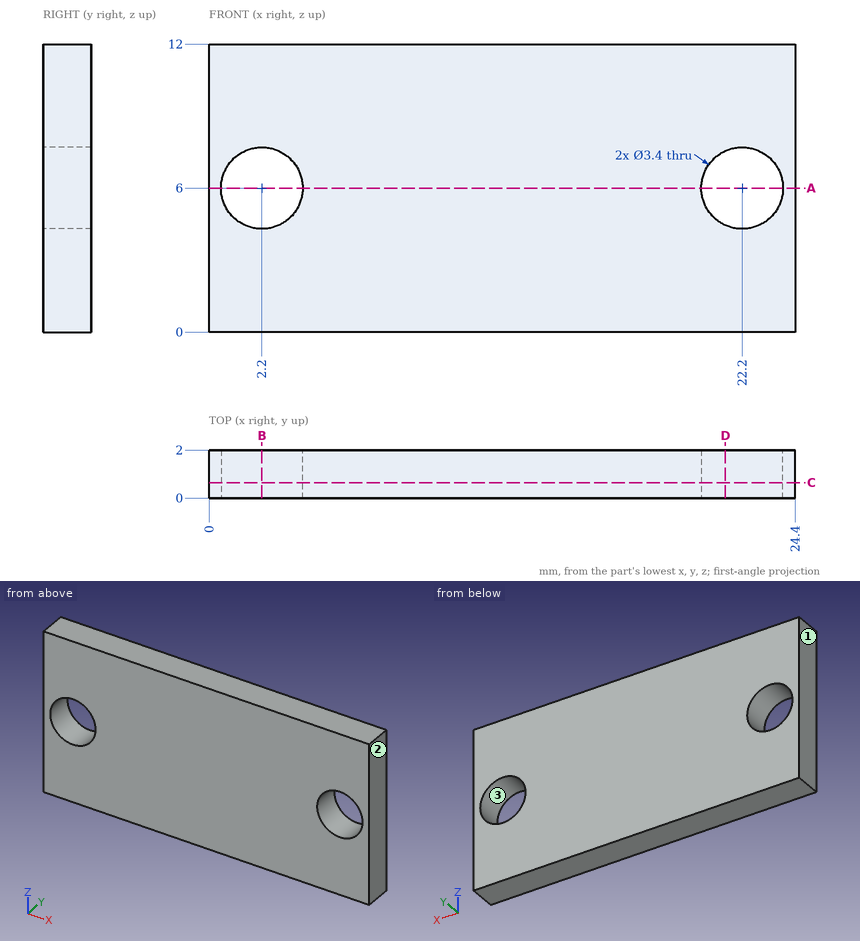
Could you check a few things on this drawing? It's one solid part, dimensions in mm from its lowest x, y, z. Give positions to 0.01 mm unless a question says otherwise; leave off trailing zeros. Write each loop counter-clockwise with the first axis right and the second up, starting at its lowest first coordinate (ties: lowest second). Pieces come first, ordered by that corner, then holes. Notation, with made-up numbers: (81.5, 19) -> (85.5, 19) arc R24 ccw to (85.5, 30) -> close; hole circle Ø1 at (59, 61.5). An arc over 180 degrees is marked (long way). Answer as a JSON object with one key per item and string values.
Q1. We'd pull the mould along X, two halves only. Please class the marked faces 1, 2 and 3: released by +X, released by -X, zero draft, split by the parting line, or undercut.
Taken from the geometry:
{"face 1": "released by -X", "face 2": "released by +X", "face 3": "undercut"}
Q2. Will this pin go through, and if not, where does the flat tip stop? pin 1 Ø2.5 at (x, z) = (22.2, 6) entering from -Y (3 decimals).
Taken from the geometry:
{"pin 1": "passes through"}
Q3. Suppose I cut it at C-C on y = 0.65. Write out the boundary of the cut face in (x, z), then the cut area to 3 significant figures.
Taken from the geometry:
{"outline": "(0, 0) -> (24.4, 0) -> (24.4, 12) -> (0, 12) -> close; hole circle Ø3.4 at (2.2, 6); hole circle Ø3.4 at (22.2, 6)", "area": "275 mm²"}
Q4. Suppose I cut it at A-A on z = 6. Write out the boundary of the cut face in (x, y).
Taken from the geometry:
{"outline": "(0, 0) -> (0.5, 0) -> (0.5, 2) -> (0, 2) -> close; (3.9, 0) -> (20.5, 0) -> (20.5, 2) -> (3.9, 2) -> close; (23.9, 0) -> (24.4, 0) -> (24.4, 2) -> (23.9, 2) -> close"}
Q5. Suppose I cut it at B-B on x = 2.2. Write out the boundary of the cut face in (y, z).
Taken from the geometry:
{"outline": "(0, 0) -> (2, 0) -> (2, 4.3) -> (0, 4.3) -> close; (0, 7.7) -> (2, 7.7) -> (2, 12) -> (0, 12) -> close"}
Q6. Please list where these lines run through material, in increasing order: L1, parallel to X at y = 0.7, z = 6; L2, parallel to Z at x = 2.2, y = 1.5; L3, parallel to X at y = 1.75, z = 7.25.
Taken from the geometry:
{"L1": "x = 0 to 0.5, 3.9 to 20.5, 23.9 to 24.4", "L2": "z = 0 to 4.3, 7.7 to 12", "L3": "x = 0 to 1.05, 3.35 to 21.05, 23.35 to 24.4"}
Q7. Suppose I cut it at D-D on x = 21.5. Write out the boundary of the cut face in (y, z), then the cut area to 3 significant figures.
Taken from the geometry:
{"outline": "(0, 0) -> (2, 0) -> (2, 4.45) -> (0, 4.45) -> close; (0, 7.55) -> (2, 7.55) -> (2, 12) -> (0, 12) -> close", "area": "17.8 mm²"}
